from build123d import *

# Parameters (mm, degrees)
SKETCH1_R           = 0.95
SKETCH1_R_2         = 0.7
BOSS_EXTRUDE1_DEPTH = 4
SKETCH2_W           = 16.2
SKETCH2_H           = 11.98
CUT_EXTRUDE1_DEPTH  = 2


with BuildPart() as part:
    # Sketch1 → Boss-Extrude1 (new body)
    with BuildSketch(Plane.XY):
        with BuildLine():
            Line((3.1, 16.98), (-3.1, 16.98))
            ThreePointArc((-3.1, 16.98), (-6.635533906, 15.515533906), (-8.1, 11.98))
            Line((-8.1, 11.98), (-8.1, 6))
            Line((-8.1, 6), (-4.1, 6))
            Line((-4.1, 6), (-4.1, 4))
            Line((-4.1, 4), (-8.1, 4))
            Line((-8.1, 4), (-8.1, 2))
            ThreePointArc((-8.1, 2), (-7.514213562, 0.585786438), (-6.1, 0))
            Line((-6.1, 0), (6.1, 0))
            ThreePointArc((6.1, 0), (7.514213562, 0.585786438), (8.1, 2))
            Line((8.1, 2), (8.1, 4))
            Line((8.1, 4), (4.1, 4))
            Line((4.1, 4), (4.1, 6))
            Line((4.1, 6), (8.1, 6))
            Line((8.1, 6), (8.1, 11.98))
            ThreePointArc((8.1, 11.98), (6.635533906, 15.515533906), (3.1, 16.98))
        make_face()
        with Locations((-5.15, 2)):
            Circle(SKETCH1_R, mode=Mode.SUBTRACT)
        with Locations((-5.1, 13.98)):
            Circle(SKETCH1_R_2, mode=Mode.SUBTRACT)
        with Locations((-5.35, 8.5)):
            Circle(SKETCH1_R, mode=Mode.SUBTRACT)
        with Locations((5.35, 8.5)):
            Circle(SKETCH1_R, mode=Mode.SUBTRACT)
        with Locations((5.1, 13.98)):
            Circle(SKETCH1_R_2, mode=Mode.SUBTRACT)
        with Locations((5.15, 2)):
            Circle(SKETCH1_R, mode=Mode.SUBTRACT)
    extrude(amount=BOSS_EXTRUDE1_DEPTH)

    # Sketch2 → Cut-Extrude1 (cut)
    with BuildSketch(Plane.XY):
        with Locations((0, 5.99)):
            Rectangle(SKETCH2_W, SKETCH2_H)
    extrude(amount=CUT_EXTRUDE1_DEPTH, mode=Mode.SUBTRACT)


solid = part.part
Here's how the part is built. I have some questions about the finished solid (model axes, mm). A direction names the side the tool comes from. Give positions to 0.01 mm unless a question says otherwise; leave off trailing zeros. Write each loop counter-clockwise with the first axis right and the second up, starting at its lowest first coordinate (ties: lowest second). Pieces come first, ordered by that corner, then holes. Notation, with made-up numbers: (3.5, -3.5) -> (28.5, -3.5) arc R18 cw to (28.5, 7.5) -> close; hole circle Ø9 at (42.5, 17). An arc over 180 degrees is marked (long way). Use one line per item in the form item = value. Start each with the question number.
1. Will these pins go through, and if not, where does the flat tip stop? pin 1 Ø1.6 at (x, z) = (5.5, 3) entering from -Y; pin 2 Ø0.6 at (y, z) = (5.5, 2.5) entering from +X; pin 3 Ø1 at (y, z) = (5, 3) entering from -X; pin 4 Ø2 at (x, y) = (-5.35, 8.5) entering from -Z.
2. Imagine slicing it at B-B on x = 5.35. List the corners of the cut face in (y, z) for me, plus the area to 3 significant figures.
3. Imagine slicing it at A-A on y = 8.5. List the corners of the cut face in (x, z) for me, plus the area to 3 significant figures.
4. If I drill on L1, parallel to X at y = 2, z = 2.8; L2, parallel to X at y = 13.75, z = 3.15; L3, parallel to Y at x = 5.35, z = 3.2, over which ranges is the centre line in solid material (lowest first)?
5. Imagine slicing it at C-C on z = 3.05. List the corners of the cut face in (x, y) for me, plus the area to 3 significant figures.
6. On a 3-axis mill with a long thin cutter (end or side, diameter ignored), from which of +Z, -Z, +X, -X, +Y, -Y can I reach the whole of each face in a straight line? I mean faces 1 (the face through (0, 6, 2)), 2 (the face through (6, 4, 3)), 3 (the face through (-6, 4, 3)). Say none if no direction works.
7. Imagine slicing it at D-D on x = -0.75. List the corners of the cut face in (y, z) for me.
8. Thinking about a two-plate mould opening in Y: for faces 4 (the face through (6.67, 15.48, 1.97)), 5 (the face through (-6, 6, 3)), 6 (the face through (-8.1, 9, 3)), which applies, +Y half, -Y half, draft (parallel to the pull), parting line (faces both ways), or undercut?
Entries:
q1.pin_1 = 0
q1.pin_2 = 4.1
q1.pin_3 = -4.1
q1.pin_4 = 2
q2.outline = (0, 2) -> (1.07, 2) -> (1.07, 4) -> (0, 4) -> close; (2.93, 2) -> (4, 2) -> (4, 4) -> (2.93, 4) -> close; (6, 2) -> (7.55, 2) -> (7.55, 4) -> (6, 4) -> close; (9.45, 2) -> (11.98, 2) -> (11.98, 0) -> (13.33, 0) -> (13.33, 4) -> (9.45, 4) -> close; (14.63, 0) -> (16.45, 0) -> (16.45, 4) -> (14.63, 4) -> close
q2.area = 25.1 mm²
q3.outline = (-8.1, 2) -> (-6.3, 2) -> (-6.3, 4) -> (-8.1, 4) -> close; (-4.4, 2) -> (4.4, 2) -> (4.4, 4) -> (-4.4, 4) -> close; (6.3, 2) -> (8.1, 2) -> (8.1, 4) -> (6.3, 4) -> close
q3.area = 24.8 mm²
q4.L1 = -8.1 to -6.1, -4.2 to 4.2, 6.1 to 8.1
q4.L2 = -7.78 to -5.76, -4.44 to 4.44, 5.76 to 7.78
q4.L3 = 0 to 1.07, 2.93 to 4, 6 to 7.55, 9.45 to 13.33, 14.63 to 16.45
q5.outline = (-8.1, 2) arc R2 ccw to (-6.1, 0) -> (6.1, 0) arc R2 ccw to (8.1, 2) -> (8.1, 4) -> (4.1, 4) -> (4.1, 6) -> (8.1, 6) -> (8.1, 11.98) arc R5 ccw to (3.1, 16.98) -> (-3.1, 16.98) arc R5 ccw to (-8.1, 11.98) -> (-8.1, 6) -> (-4.1, 6) -> (-4.1, 4) -> (-8.1, 4) -> close; hole circle Ø1.9 at (-5.35, 8.5); hole circle Ø1.9 at (-5.15, 2); hole circle Ø1.4 at (-5.1, 13.98); hole circle Ø1.9 at (5.15, 2); hole circle Ø1.9 at (5.35, 8.5); hole circle Ø1.4 at (5.1, 13.98)
q5.area = 232 mm²
q6.face_1 = -Z, +X, -X, -Y
q6.face_2 = +Z, -Z, +X
q6.face_3 = +Z, -Z, -X
q7.outline = (0, 2) -> (11.98, 2) -> (11.98, 0) -> (16.98, 0) -> (16.98, 4) -> (0, 4) -> close
q8.face_4 = +Y half
q8.face_5 = undercut
q8.face_6 = draft
